For this review, take the finished solid that the model builds, in its own axes (mm). A direction names the side the tool comes from. Give positions to 0.01 mm unless a question says otherwise; leave off trailing zeros. Loops run counter-clockwise (first coordinate to the right, second up) from the corner with the lowest first, then second, coordinate; pieces in that order, holes last.
```python
from build123d import *

# Parameters (mm, degrees)
SKETCH1_W           = 50
SKETCH1_H           = 30
BOSS_EXTRUDE1_DEPTH = 3
SKETCH2_R           = 1.75
CUT_EXTRUDE1_DEPTH  = 4
SKETCH3_W           = 30
SKETCH3_H           = 20
BOSS_EXTRUDE2_DEPTH = 5
BOSS_EXTRUDE3_DEPTH = 30
SKETCH5_R           = 4
CUT_EXTRUDE2_DEPTH  = 20
SKETCH6_W           = 50
SKETCH6_H           = 8
CUT_EXTRUDE3_DEPTH  = 20
SKETCH7_W           = 3
SKETCH7_H           = 22
BOSS_EXTRUDE4_DEPTH = 3
SKETCH8_W           = 3
SKETCH8_H           = 22
BOSS_EXTRUDE5_DEPTH = 22
SKETCH9_R           = 1.75
CUT_EXTRUDE4_DEPTH  = 54
SKETCH10_W          = 23
SKETCH10_H          = 22
SKETCH10_R          = 1.75
BOSS_EXTRUDE6_DEPTH = 1
SKETCH11_W          = 26
SKETCH11_H          = 22
SKETCH11_R          = 1.75
BOSS_EXTRUDE7_DEPTH = 1
FILLET1_R           = 2


with BuildPart() as part:
    # Sketch1 → Boss-Extrude1 (new body)
    with BuildSketch(Plane.XY):
        with Locations((25, 15)):
            Rectangle(SKETCH1_W, SKETCH1_H)
    extrude(amount=BOSS_EXTRUDE1_DEPTH)

    # Sketch2 → Cut-Extrude1 (cut, through all)
    with BuildSketch(Plane.XY.offset(3)):
        with Locations((38, 7.5)):
            Circle(SKETCH2_R)
    extrude(amount=-CUT_EXTRUDE1_DEPTH, mode=Mode.SUBTRACT)

    # Sketch3 → Boss-Extrude2 (add)
    with BuildSketch(Plane.XY.offset(3)):
        with Locations((15, 12)):
            Rectangle(SKETCH3_W, SKETCH3_H)
    extrude(amount=BOSS_EXTRUDE2_DEPTH)

    # Sketch4 → Boss-Extrude3 (add)
    with BuildSketch(Plane.ZY):
        with BuildLine():
            Line((8, 4.5), (8, 19.5))
            ThreePointArc((8, 19.5), (15.5, 12), (8, 4.5))
        make_face()
    extrude(amount=-BOSS_EXTRUDE3_DEPTH)

    # Sketch5 → Cut-Extrude2 (cut)
    with BuildSketch(Plane.ZY):
        with Locations((8, 12)):
            Circle(SKETCH5_R)
    extrude(amount=-CUT_EXTRUDE2_DEPTH, mode=Mode.SUBTRACT)

    # Sketch6 → Cut-Extrude3 (cut)
    with BuildSketch(Plane.XY.offset(3)):
        with Locations((25, 26)):
            Rectangle(SKETCH6_W, SKETCH6_H)
    extrude(amount=-CUT_EXTRUDE3_DEPTH, mode=Mode.SUBTRACT)

    # Sketch7 → Boss-Extrude4 (add)
    with BuildSketch(Plane(origin=(50, 0, 0), x_dir=(0, 0, -1), z_dir=(1, 0, 0))):
        with Locations((-1.5, 11)):
            Rectangle(SKETCH7_W, SKETCH7_H)
    extrude(amount=BOSS_EXTRUDE4_DEPTH)

    # Sketch8 → Boss-Extrude5 (add)
    with BuildSketch(Plane(origin=(0, 0, 0), x_dir=(-1, 0, 0), z_dir=(0, 0, -1))):
        with Locations((-51.5, 11)):
            Rectangle(SKETCH8_W, SKETCH8_H)
    extrude(amount=BOSS_EXTRUDE5_DEPTH)

    # Sketch9 → Cut-Extrude4 (cut, through all)
    with BuildSketch(Plane(origin=(53, 0, 0), x_dir=(0, 0, -1), z_dir=(1, 0, 0))):
        with Locations((12, 7.5)):
            Circle(SKETCH9_R)
    extrude(amount=-CUT_EXTRUDE4_DEPTH, mode=Mode.SUBTRACT)

    # Sketch10 → Boss-Extrude6 (add)
    with BuildSketch(Plane.XY.offset(3)):
        with Locations((41.5, 11)):
            Rectangle(SKETCH10_W, SKETCH10_H)
        with Locations((38, 7.5)):
            Circle(SKETCH10_R, mode=Mode.SUBTRACT)
    extrude(amount=BOSS_EXTRUDE6_DEPTH)

    # Sketch11 → Boss-Extrude7 (add)
    with BuildSketch(Plane(origin=(53, 0, 0), x_dir=(0, 0, -1), z_dir=(1, 0, 0))):
        with Locations((9, 11)):
            Rectangle(SKETCH11_W, SKETCH11_H)
        with Locations((12, 7.5)):
            Circle(SKETCH11_R, mode=Mode.SUBTRACT)
    extrude(amount=BOSS_EXTRUDE7_DEPTH)

    # Fillet1
    fillet1_edges = [part.edges().sort_by_distance(p)[0] for p in [
        (30, 12, 4),
        (54, 11, 4),
    ]]
    fillet(fillet1_edges, radius=FILLET1_R)


solid = part.part
```
Item 1: Take a section at B-B on z = -12. Give the boundary of the cut face in (x, y).
Answer:
outline: (50, 0) - (54, 0) - (54, 5.75) - (50, 5.75) - close; (50, 9.25) - (54, 9.25) - (54, 22) - (50, 22) - close
Item 2: Take a section at D-D on x = 8.5. Give the boundary of the cut face in (y, z).
Answer:
outline: (0, 0) - (22, 0) - (22, 8) - (19.5, 8) arc R7.5 ccw to (4.5, 8) - (2, 8) - (2, 3) - (0, 3) - close; hole circle Ø8 at (12, 8)
Item 3: The part is to be moulded in two halves that separate along Z. For faces 1 (the flat face through (54, 11, -10)), 2 (the flat face through (15, 1, 3)), 3 (the flat face through (52, 11, -22)), 4 (the flat face through (20, 12, 8)), say which applies: released by +Z, released by -Z, zero draft, split by the parting line, or undercut.
Answer:
face 1: zero draft
face 2: released by +Z
face 3: released by -Z
face 4: undercut
Item 4: Take a section at A-A on x = 38. Give the boundary of the cut face in (y, z).
Answer:
outline: (0, 0) - (5.75, 0) - (5.75, 4) - (0, 4) - close; (9.25, 0) - (22, 0) - (22, 4) - (9.25, 4) - close
Item 5: Tool access review of faces 5 (the flat face through (50, 11, -11)), 6 (the flat face through (15, 21, 8)), 7 (the cylindrical face through (9.86, 14.7, 5.05)): name each direction out of +Z, -Z, +X, -X, +Y, -Y from which nothing blocks a thin tool from reaching the whole face with its end or side.
Answer:
face 5: -Z, -X, +Y, -Y
face 6: +Z, +X, -X, +Y
face 7: -X
Item 6: For L1, parallel to Y at x = 53.55, z = -12; L2, parallel to Z at x = 43, y = 15.25; L3, parallel to Y at x = 18.5, z = 5, list the stretches that pass through material, from the lowest coordinate up.
Answer:
L1: y = 0 to 5.75, 9.25 to 22
L2: z = 0 to 4
L3: y = 2 to 9.35, 14.65 to 22
Item 7: Take a section at C-C on y = 3.25. Give the boundary of the cut face in (x, z), and give its area (3 significant figures).
Answer:
outline: (0, 0) - (50, 0) - (50, -22) - (54, -22) - (54, 2) arc R2 ccw to (52, 4) - (32, 4) arc R2 cw to (30, 6) - (30, 8) - (0, 8) - close
area: 424 mm2
Item 8: Clearance check with flat-ended pins moving along their axes: pin 1 Ø5.5 at (x, y) = (38, 7.5) entering from -Z; pin 2 Ø9 at (y, z) = (12, 8) entering from +X; pin 3 Ø2 at (x, z) = (8.5, 7.5) entering from -Y; pin 4 Ø6.5 at (y, z) = (10.5, 10) entering from -X. State where each tip first meets the part, or that it passes through.
Answer:
pin 1: stops at z = 0
pin 2: stops at x = 53.32
pin 3: stops at y = 2
pin 4: stops at x = 0
